CAD build for the part. Positions are in the model's coordinates, mm. Face numbers are marked on the shaded views. Coordinates: 2 decimals unless noted, no trailing zeros. Write each loop counter-clockwise with the first axis right and the second up, starting at its lowest first coordinate (ties: lowest second). Pieces come first, ordered by that corner, then holes. Notation, with made-up numbers: (64.25, -6.75) - (81.25, -6.75) arc R28 ccw to (81.25, 27.25) - close; hole circle Ø9 at (-2, 78.5). An arc over 180 degrees is marked (long way). One line per question, with ' | ' between items. Start each with the question number.
1. Probe line 1 (Y direction, x = 0, z = 1.9); line 2 (Y direction, x = -0.25, z = 0.85); line 3 (X direction, y = -3, z = 2.7). List the from-to ranges inside material, lowest first.
2. Two-plate mould, pull along X, no slides. Class the marked faces 1, 2 and 3: +X half, -X half, draft (parallel to the pull), parting line (faces both ways), or undercut.
3. Flat gauge pins, fed straight in: P1, Ø6, axis at x = 0, y = 9.779, coming from the +Z side (3 decimals); P2, Ø1, axis at x = 7.5, z = 2, coming from the +Y side. Where does each tip first touch, or does it go through?
4. Band-saw the part on C-C, the plane x = 8.5. Write the cut outline in (y, z) (3 decimals), then the cut area to 3 significant figures.
5. Band-saw the part on A-A, the plane x = 0. Write the cut outline in (y, z) (3 decimals).
6. Band-saw the part on D-D, the plane y = -4.25. Write the cut outline in (x, z) (3 decimals), then the cut area to 3 significant figures.
7. Band-saw the part on B-B, the plane y = 0. Write the cut outline in (x, z) (3 decimals), then the cut area to 3 significant figures.
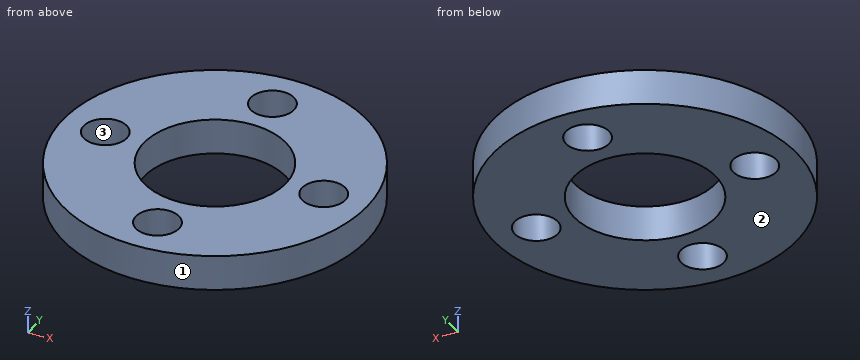
Autodesk Inventor part; units mm, degrees
ref_plane "YZ Plane" through (0, 0, 0) normal (1, 0, 0) x (0, 1, 0)
ref_plane "XZ Plane" through (0, 0, 0) normal (0, 1, 0) x (-1, 0, 0)
ref_plane "XY Plane" through (0, 0, 0) normal (0, 0, 1) x (1, 0, 0)
ref_plane "Work Plane1" through (0, 0, 0) normal (0, 0, 1) x (1, 0, 0)
sketch "Sketch1" plane through (0, 0, 0) normal (0, 0, 1) x (1, 0, 0)
  arc A0 (-12.3389, 9.6089) -> (-9.6089, 12.3389) centre (-10.9739, 10.9739) ccw construction
  circle A1 centre (0, 9.779) radius 1.9304
  circle A2 centre (9.6987, 0) radius 1.9304
  circle A3 centre (0, -9.779) radius 1.9304
  circle A4 centre (-9.779, 0) radius 1.9304
  circle A5 centre (0, 0) radius 6.35
  circle A6 centre (0, 0) radius 13.589
extrude "Extrusion1" add sketch "Sketch1" along normal blind 3.175
properties part number "spool 4in inner plate"
Filled in:
1) line 1: y = -13.59 to -11.71, -7.85 to -6.35, 6.35 to 7.85, 11.71 to 13.59 | line 2: y = -13.59 to -11.69, -7.86 to -6.35, 6.35 to 7.86, 11.69 to 13.59 | line 3: x = -13.25 to -5.6, 5.6 to 13.25
2) face 1: parting line | face 2: draft | face 3: undercut
3) P1: stops at z = 3.175 | P2: stops at y = 11.65
4) outline: (-10.602, 0) - (-1.513, 0) - (-1.513, 3.175) - (-10.602, 3.175) - close; (1.513, 0) - (10.602, 0) - (10.602, 3.175) - (1.513, 3.175) - close | area: 57.7 mm²
5) outline: (-13.589, 0) - (-11.709, 0) - (-11.709, 3.175) - (-13.589, 3.175) - close; (-7.849, 0) - (-6.35, 0) - (-6.35, 3.175) - (-7.849, 3.175) - close; (6.35, 0) - (7.849, 0) - (7.849, 3.175) - (6.35, 3.175) - close; (11.709, 0) - (13.589, 0) - (13.589, 3.175) - (11.709, 3.175) - close
6) outline: (-12.907, 0) - (-4.718, 0) - (-4.718, 3.175) - (-12.907, 3.175) - close; (4.718, 0) - (12.907, 0) - (12.907, 3.175) - (4.718, 3.175) - close | area: 52.0 mm²
7) outline: (-13.589, 0) - (-11.709, 0) - (-11.709, 3.175) - (-13.589, 3.175) - close; (-7.849, 0) - (-6.35, 0) - (-6.35, 3.175) - (-7.849, 3.175) - close; (6.35, 0) - (7.768, 0) - (7.768, 3.175) - (6.35, 3.175) - close; (11.629, 0) - (13.589, 0) - (13.589, 3.175) - (11.629, 3.175) - close | area: 21.5 mm²
